Source: CAD feature listing. Evaluate the final solid. Frame: model axes, mm. A direction names the side the tool comes from. Coordinates: 2 decimals unless noted, no trailing zeros. Write each loop counter-clockwise with the first axis right and the second up, starting at its lowest first coordinate (ties: lowest second). Pieces come first, ordered by that corner, then holes. Notation, with made-up numbers: M 79,74.5 L 99,74.5 A35 ccw 99,106.5 Z; hole C 77,23.25 d6. An arc over 180 degrees is marked long. One line per item, written item: value. Start each with the question number.
Item 1: Cut plane A-A, the plane x = 20. Output: boundary loops of the cut face in (y, z), then the cut area to 3 significant figures.
Item 2: Mould query, pull axis Z, two halves, no side actions, for faces 3 (the flat face through (8, 5, 85)), 4 (the flat face through (0, 20, 42)), 5 (the cylindrical face through (19.09, 2.46, 71.94)), 6 (the cylindrical face through (14.445, 2.465, 15.741)). Classes: released by +Z, released by -Z, zero draft, split by the parting line, or undercut.
Item 3: Cut plane C-C, the plane z = 47.5. Output: boundary loops of the cut face in (x, y).
Item 4: Ray query, L1, parallel to Z at x = 20, y = 2.75; L2, parallel to Z at x = 23, y = 4; L3, parallel to Y at x = 21, z = 30. Return the intervals inside material, ascending. Write a range as from..to.
Item 5: Set-up query: faces 1 (the flat face through (5, 24, 42)), 2 (the flat face through (1, 40, 42)). Return all of +Z, -Z, +X, -X, +Y, -Y with unobstructed straight access to the full face (end or side cutting, diameter ignored); none if empty.
Item 6: Cut plane D-D, the plane y = 13.5. Output: boundary loops of the cut face in (x, z).
Item 7: Pin query (flat end, axial travel): P1, Ø8, axis at y = 34.5, z = 64.5, coming from the +X side; P2, Ø8, axis at x = 26.5, z = 31.5, coming from the +Y side. Return the tip coordinate at first contact, or that it passes through.
Item 8: Cut plane B-B, the plane z = 65. Output: boundary loops of the cut face in (x, y).
```python
from build123d import *

# Parameters (mm, degrees)
F1_DEPTH = 85
F2_R     = 7
F3_DEPTH = 40.001


with BuildPart() as f1:
    # F0 (on Top) → F1 (new body)
    with BuildSketch(Plane.XY):
        with BuildLine():
            Line((0, 40), (0, 0))
            Line((0, 0), (40, 0))
            Line((40, 0), (40, 2.6))
            ThreePointArc((40, 2.6), (39.297056, 4.297056), (37.6, 5))
            Line((37.6, 5), (11, 5))
            ThreePointArc((11, 5), (6.757359, 6.757359), (5, 11))
            Line((5, 11), (5, 37.6))
            ThreePointArc((5, 37.6), (4.297056, 39.297056), (2.6, 40))
            Line((2.6, 40), (0, 40))
        make_face()
    extrude(amount=F1_DEPTH)

    # F2 (on face) → F3 (cut, through all)
    with BuildSketch(Plane.XZ):
        with Locations((20, 65)):
            Circle(F2_R)
        with Locations((20, 20)):
            Circle(F2_R)
    extrude(amount=-F3_DEPTH, mode=Mode.SUBTRACT)


solid = f1.part
```
From the geometry:
1. outline: M 0,0 L 5,0 L 5,13 L 0,13 Z; M 0,27 L 5,27 L 5,58 L 0,58 Z; M 0,72 L 5,72 L 5,85 L 0,85 Z
1. area: 285 mm²
2. face 3: released by +Z
2. face 4: zero draft
2. face 5: undercut
2. face 6: undercut
3. outline: M 0,0 L 40,0 L 40,2.6 A2.4 ccw 37.6,5 L 11,5 A6 cw 5,11 L 5,37.6 A2.4 ccw 2.6,40 L 0,40 Z
4. L1: z = 0..13, 27..58, 72..85
4. L2: z = 0..13.68, 26.32..58.68, 71.32..85
4. L3: y = 0..5
5. face 1: +Z, -Z, +X, +Y
5. face 2: +Z, -Z, +X, -X, +Y
6. outline: M 0,0 L 5,0 L 5,85 L 0,85 Z
7. P1: stops at x = 5
7. P2: stops at y = 5
8. outline: M 0,0 L 13,0 L 13,5 L 11,5 A6 cw 5,11 L 5,37.6 A2.4 ccw 2.6,40 L 0,40 Z; M 27,0 L 40,0 L 40,2.6 A2.4 ccw 37.6,5 L 27,5 Z
